```python
from build123d import *

# Parameters (mm, degrees)
EXTRUDE_THIN1_DEPTH = 5
SKETCH5_W           = 26.389754353
SKETCH5_H           = 10
BOSS_EXTRUDE1_DEPTH = 0.1
SKETCH6_R           = 4
BOSS_EXTRUDE2_DEPTH = 12
CHAMFER1_SIZE       = 2
CHAMFER1_SIZE2      = 0.932615316
FILLET1_R           = 2


with BuildPart() as part:
    # Sketch3 → Extrude-Thin1 (new body, symmetric)
    with BuildSketch(Plane(origin=(0, 0, 0), x_dir=(1, 0, 0), z_dir=(0, 1, 0))):
        with BuildLine():
            Line((16.248076809, 30), (16.248076809, 0))
            ThreePointArc((16.248076809, 0), (0, -16.248076809), (-16.248076809, 0))
            Line((-16.248076809, 0), (-16.248076809, 30))
            Line((-16.248076809, 30), (-16.148076809, 30))
            Line((-16.148076809, 30), (-16.148076809, 0))
            ThreePointArc((-16.148076809, 0), (0, -16.148076809), (16.148076809, 0))
            Line((16.148076809, 0), (16.148076809, 30))
            Line((16.148076809, 30), (16.248076809, 30))
        make_face()
    extrude(amount=EXTRUDE_THIN1_DEPTH, both=True)

    # Sketch5 → Boss-Extrude1 (add)
    with BuildSketch(Plane.ZY.offset(16.248076809)):
        with Locations((-13.194877177, 0)):
            Rectangle(SKETCH5_W, SKETCH5_H)
    extrude(amount=-BOSS_EXTRUDE1_DEPTH)

    # Sketch6 → Boss-Extrude2 (add)
    with BuildSketch(Plane(origin=(16.248076809, 0, 0), x_dir=(0, 0, -1), z_dir=(1, 0, 0))):
        with Locations((20, 0)):
            Circle(SKETCH6_R)
    extrude(amount=BOSS_EXTRUDE2_DEPTH)

    # Chamfer1
    chamfer1_edges = [part.edges().sort_by_distance(p)[0] for p in [
        (28.248076809, 0, -16),
    ]]
    chamfer1_side = [part.faces().sort_by_distance(p)[0] for p in [
        (22.248076809, 0, -16),
    ]]
    chamfer(chamfer1_edges, length=CHAMFER1_SIZE, length2=CHAMFER1_SIZE2, reference=chamfer1_side[0])

    # Fillet1
    fillet1_edges = [part.edges().sort_by_distance(p)[0] for p in [
        (28.248076809, 0, -16.932615316),
        (26.248076809, 0, -16),
    ]]
    fillet(fillet1_edges, radius=FILLET1_R)


solid = part.part
```
The listing builds one solid part. Answer for the finished solid, in the listing's coordinates (mm). A direction names the side the tool comes from. Round coordinates to 2 decimals unless told otherwise and drop trailing zeros. Loops run counter-clockwise (first coordinate to the right, second up) from the corner with the lowest first, then second, coordinate; pieces in that order, holes last. Notation, with made-up numbers: (74, 18) - (94, 18) arc R32 cw to (94, 48) - close; hole circle Ø9 at (-22, 39). An arc over 180 degrees is marked (long way). Use one line per item in the form item = value. Start each with the question number.
1. Consider line 1 (Z direction, x = 23.5, y = -0.25); line 2 (Z direction, x = 19, y = -1). Determine where each line is inside the solid, lowest interval first. Write a range as [from, to].
2. The part is cut by section C-C on x = 17. Determine the outline of the cut face in (y, z), then the cut area to 3 significant figures.
3. The part is cut by section A-A on z = -10. Determine the outline of the cut face in (x, y).
4. A tool of negligible diameter and unlimited length cuts with its end or side. For faces 1 (the face through (20.96, 2.7, -17.05)), 2 (the face through (28.248, 0, -20)), from which of +Z, -Z, +X, -X, +Y, -Y can it reach the whole face along a straight path? Write none if from no direction.
5. The part is cut by section B-B on z = 13. Determine the outline of the cut face in (x, y).
6. The part is cut by section D-D on x = 0. Determine the outline of the cut face in (y, z).
7. Given pin 1 Ø2 at (y, z) = (-2, 10.5) entering from +X; pin 2 Ø1 at (x, y) = (11.5, 1) entering from +Z; pin 3 Ø3 at (y, z) = (0.5, -8) entering from +X, each flat-ended and moving along its own axis, determine where each tip first touches the part or whether it passes through.
Geometry check:
q1.line_1 = [-23.99, -16.01]
q1.line_2 = [-23.87, -16.13]
q2.outline = circle Ø8 at (0, -20)
q2.area = 50.3 mm^2
q3.outline = (-16.25, -5) - (-16.15, -5) - (-16.15, 5) - (-16.25, 5) - close; (16.15, -5) - (16.25, -5) - (16.25, 5) - (16.15, 5) - close
q4.face_1 = +X
q4.face_2 = +Z, -Z, +X, +Y, -Y
q5.outline = (-9.75, -5) - (-9.58, -5) - (-9.58, 5) - (-9.75, 5) - close; (9.58, -5) - (9.75, -5) - (9.75, 5) - (9.58, 5) - close
q6.outline = (-5, 16.15) - (5, 16.15) - (5, 16.25) - (-5, 16.25) - close
q7.pin_1 = 13.18
q7.pin_2 = 11.96
q7.pin_3 = 16.25
